Autodesk Inventor part; units mm, degrees
ref_plane "YZ Plane" through (0, 0, 0) normal (1, 0, 0) x (0, 1, 0)
ref_plane "XZ Plane" through (0, 0, 0) normal (0, 1, 0) x (-1, 0, 0)
ref_plane "XY Plane" through (0, 0, 0) normal (0, 0, 1) x (1, 0, 0)
sketch "Sketch1" plane through (0, 0, 0) normal (0, 0, 1) x (1, 0, 0)
  line L0 (0, 0) -> (153.9875, 0)
  line L1 (153.9875, 0) -> (153.9875, 101.6)
  line L2 (153.9875, 101.6) -> (0, 101.6)
  line L3 (0, 101.6) -> (0, 0)
  dimension "d0" = 153.9875
  dimension "d1" = 101.6
extrude "Extrusion1" add sketch "Sketch1" along normal blind 38.1
sketch "Sketch2" plane through (0, 101.6, 0) normal (0, 1, 0) x (1, 0, 0)
  line L0 (0, -38.1) -> (153.9875, -38.1)
  line L1 (0, 0) -> (0, -38.1)
  circle A0 centre (31.75, -19.05) radius 10.4767
  dimension "d4" = 31.75
  dimension "d5" = 19.05
extrude "Extrusion2" cut sketch "Sketch2" against normal blind 6.35
sketch "Sketch3" plane through (0, 0, 38.1) normal (0, 0, 1) x (1, 0, 0)
  line L0 (0, 0) -> (0, 101.6)
  line L1 (0, 101.6) -> (153.9875, 101.6)
  circle A0 centre (87.63, 50.8) radius 3.175
  dimension "d8" = 6.35
  dimension "d9" = 87.63
  dimension "d10" = 50.8
extrude "Extrusion3" cut sketch "Sketch3" against normal blind 9.525
sketch "Sketch4" plane through (0, 0, 38.1) normal (0, 0, 1) x (1, 0, 0)
  line L0 (42.2267, 95.25) -> (21.2733, 95.25)
  line L1 (31.75, 95.25) -> (31.75, 50.8) construction
  circle A0 centre (31.75, 86.77) radius 1.27
  dimension "d13" = 2.54
extrude "Extrusion4" cut sketch "Sketch4" against normal blind 25.4
properties part number "aaxaProjector01" material "ABS Plastic"
Geometry check sheet. Reference: the model listing, model coordinates, mm. A direction names the side the tool comes from. Give positions to 0.01 mm unless a question says otherwise; leave off trailing zeros. Order: outer loops, then holes, each group sorted by start corner. A loop starts at its lowest first (then second) coordinate and runs counter-clockwise, first axis right, second up. Notation, with made-up numbers: M -22,74 L 4,74 A14 cw 4,86 Z; hole C 2.5,65.5 d3. An arc over 180 degrees is marked long. Use a Markdown table: item, result.
Item 1: Material ranges on line 1 along X through (y, z) = (98, 19.05); line 2 along Y through (x, z) = (87.63, 32.75) (3 decimals); line 3 along Z through (x, y) = (31.75, 99), recorded low to high.
Answers follow:
| item | result |
|---|---|
| line 1 | x = 0 to 21.27, 42.23 to 153.99 |
| line 2 | y = 0 to 47.625, 53.975 to 101.6 |
| line 3 | z = 0 to 8.57, 29.53 to 38.1 |
Item 2: Section check A-A (x = 87.63). Record the cut outline in (y, z) (3 decimals), and give its area (3 significant figures).
Answers follow:
| item | result |
|---|---|
| outline | M 0,0 L 101.6,0 L 101.6,38.1 L 53.975,38.1 L 53.975,28.575 L 47.625,28.575 L 47.625,38.1 L 0,38.1 Z |
| area | 3,810 mm2 |
Item 3: Draft check along X on faces 4 (the cylindrical face through (23.436, 98.469, 25.425)), 5 (the flat face through (153.988, 50, 19)), 6 (the flat face through (76, 52, 0)). Enter one of: +X half, -X half, draft (parallel to the pull), parting line (faces both ways), or undercut.
Answers follow:
| item | result |
|---|---|
| face 4 | undercut |
| face 5 | +X half |
| face 6 | draft |
Item 4: Tool access check on faces 1 (the cylindrical face through (89.3, 53.5, 33.4)), 2 (the flat face through (76, 52, 38.1)), 3 (the flat face through (32, 95.25, 19)). Record the directions out of +Z, -Z, +X, -X, +Y, -Y that give a thin tool (end or side, any length) a straight path to the whole face; none if there is none.
Answers follow:
| item | result |
|---|---|
| face 1 | +Z |
| face 2 | +Z, +X, -X, +Y, -Y |
| face 3 | +Y |
Item 5: Depth check by flat-ended pin: P1, Ø4, axis at x = 87.63, y = 50.8, coming from the +Z side (3 decimals); P2, Ø3, axis at x = 86.5, y = 49.5, coming from the +Z side; P3, Ø10.5, axis at x = 30.5, z = 22.5, coming from the +Y side. Enter the tip coordinate at first touch or a pass-through.
Answers follow:
| item | result |
|---|---|
| P1 | stops at z = 28.575 |
| P2 | stops at z = 38.1 |
| P3 | stops at y = 95.25 |
